Read the model definition and answer for the solid it produces. Units are mm, in the model's axes. Face numbers are marked on the shaded views. A direction names the side the tool comes from. Give positions to 0.01 mm unless a question says otherwise; leave off trailing zeros. Loops run counter-clockwise (first coordinate to the right, second up) from the corner with the lowest first, then second, coordinate; pieces in that order, holes last.
(1) Which of the six approach directions +Z, -Z, +X, -X, +Y, -Y give full straight-line access (tool end or side, diameter ignored) to the marked faces 1 and 2?
(2) Find section C-C, the plane y = 7.5. Write down the section's boundary in (x, z), then the cut area to 3 significant figures.
(3) Each of these flat-tipped pins is pushed along its axis until it touches: P1, Ø1, axis at x = 12.5, y = -0.5, coming from the -Z side; P2, Ø2, axis at y = -13.5, z = 4, coming from the -X side. Where does it stop, or does it pass through?
(4) Determine the mould class of the marked faces 3, 4, 5 and 6 for opening direction Z: pulls with the +Z half, pulls with the -Z half, needs draft (parallel to the pull), parting line crosses it, or undercut.
(5) Find section A-A, the plane z = 0. Write down the section's boundary in (x, y).
(6) Find section B-B, the plane x = -1. Write down the section's boundary in (y, z).
(7) Straight lines are drawn through the part: probe 1 along Z at (x, y) = (-8.5, 1); probe 2 along X at (y, z) = (11.5, -1.25); probe 3 along X at (y, z) = (-14, -3). For each, find the intervals that lie inside material, in ascending order.
Autodesk Inventor part; units mm, degrees
ref_plane "YZ Plane" through (0, 0, 0) normal (1, 0, 0) x (0, 1, 0)
ref_plane "XZ Plane" through (0, 0, 0) normal (0, 1, 0) x (-1, 0, 0)
ref_plane "XY Plane" through (0, 0, 0) normal (0, 0, 1) x (1, 0, 0)
sketch "Skizze1" plane through (0, 0, 0) normal (0, 1, 0) x (-1, 0, 0)
  line L0 (12.8, 3.1) -> (-12.8, 3.1)
  line L1 (-13.6, 2.3) -> (-13.6, -2.3)
  line L2 (-12.8, -3.1) -> (12.8, -3.1)
  line L3 (13.6, -2.3) -> (13.6, 2.3)
  line L4 (13.6, 3.1) -> (-13.6, -3.1) construction
  line L5 (-13.6, 3.1) -> (13.6, -3.1) construction
  arc A0 (13.6, 2.3) -> (12.8, 3.1) centre (12.8, 2.3) ccw
  arc A1 (12.8, -3.1) -> (13.6, -2.3) centre (12.8, -2.3) ccw
  arc A2 (-13.6, -2.3) -> (-12.8, -3.1) centre (-12.8, -2.3) ccw
  arc A3 (-12.8, 3.1) -> (-13.6, 2.3) centre (-12.8, 2.3) ccw
  line L6 (9.5, 0) -> (-9.5, 0) construction
  line L7 (9.5, -7.5) -> (-9.5, -7.5)
  line L8 (-9.5, 7.5) -> (9.5, 7.5)
  arc A4 (9.5, -7.5) -> (9.5, 7.5) centre (9.5, 0) ccw
  arc A5 (-9.5, 7.5) -> (-9.5, -7.5) centre (-9.5, 0) ccw
  point P0 (0, 0)
  dimension "d0" = 27.2
  dimension "d1" = 6.2
  dimension "d2" = 0.8
  dimension "d6" = 4.4
  dimension "d7" = 34
extrude "Extrusion1" add sketch "Skizze1" along normal mid plane 46.3
properties part number "Kupferspule" material "Kupfer"
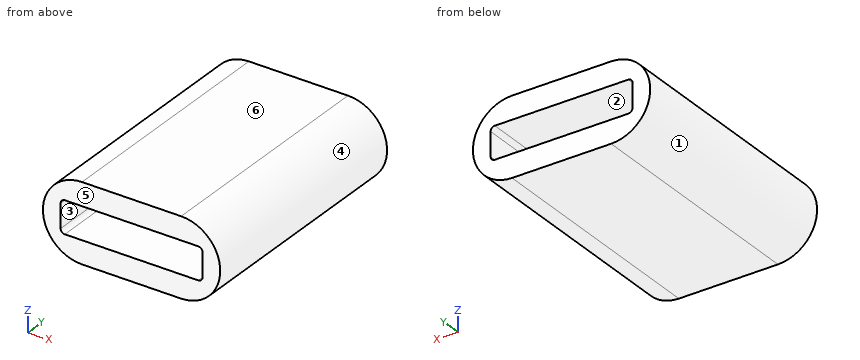
Entries:
1. face 1: -X, +Y, -Y
1. face 2: +Y, -Y
2. outline: (-9.5, -7.5) - (9.5, -7.5) arc R7.5 ccw to (9.5, 7.5) - (-9.5, 7.5) arc R7.5 ccw to start; hole (-13.6, -2.3) arc R0.8 ccw to (-12.8, -3.1) - (12.8, -3.1) arc R0.8 ccw to (13.6, -2.3) - (13.6, 2.3) arc R0.8 ccw to (12.8, 3.1) - (-12.8, 3.1) arc R0.8 ccw to (-13.6, 2.3) - close
2. area: 294 mm2
3. P1: stops at z = -7.07
3. P2: stops at x = -16.37
4. face 3: undercut
4. face 4: parting line crosses it
4. face 5: needs draft
4. face 6: pulls with the +Z half
5. outline: (-17, -23.15) - (-13.6, -23.15) - (-13.6, 23.15) - (-17, 23.15) - close; (13.6, -23.15) - (17, -23.15) - (17, 23.15) - (13.6, 23.15) - close
6. outline: (-23.15, -7.5) - (23.15, -7.5) - (23.15, -3.1) - (-23.15, -3.1) - close; (-23.15, 3.1) - (23.15, 3.1) - (23.15, 7.5) - (-23.15, 7.5) - close
7. probe 1: z = -7.5 to -3.1, 3.1 to 7.5
7. probe 2: x = -16.9 to -13.6, 13.6 to 16.9
7. probe 3: x = -16.37 to -13.19, 13.19 to 16.37
